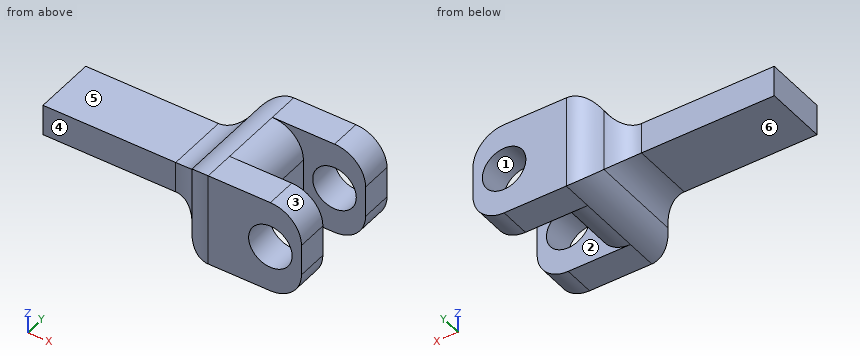
```python
from build123d import *

# Parameters (mm, degrees)
F1_DEPTH = 7.5
F3_D     = 7
F4_R     = 5
F5_R     = 4.99999
F6_W     = 10
F6_H     = 5
F7_DEPTH = 25
F8_R     = 5


# Not quite as in the source:
# - a fillet or chamfer is up to 0.001 mm smaller than in the source, because OpenCascade refuses the exact size


with BuildPart() as f1:
    # F0 (on Top) → F1 (new body, symmetric)
    with BuildSketch(Plane.XY):
        Polygon((10, 10), (-10, 10), (-10, -10), (10, -10), (10, -5), (0, -5), (0, 5), (10, 5), align=None)
    extrude(amount=F1_DEPTH, both=True)

    # F3 (through all)
    with Locations(Plane(origin=(0, 10, 0), x_dir=(-1, 0, 0), z_dir=(0, 1, 0))):
        with Locations((-5, 0)):
            Hole(F3_D / 2)

    # F4
    f4_edges = [f1.edges().sort_by_distance(p)[0] for p in [
        (10, 7.5, 7.5),
        (10, 7.5, -7.5),
        (10, -7.5, 7.5),
        (10, -7.5, -7.5),
        (-10, 10, 0),
        (-10, 0, -7.5),
        (-10, -10, 0),
        (-10, 0, 7.5),
    ]]
    fillet(f4_edges, radius=F4_R)

    # F5 (radius 5 in the source; OpenCascade refuses exactly that, so slightly less here)
    f5_edges = [f1.edges().sort_by_distance(p)[0] for p in [
        (0, 0, 7.5),
        (0, 0, -7.5),
    ]]
    fillet(f5_edges, radius=F5_R)

    # F6 (on face) → F7 (join)
    with BuildSketch(Plane(origin=(-10, 0, 0), x_dir=(0, -1, 0), z_dir=(-1, 0, 0))):
        Rectangle(F6_W, F6_H)
    extrude(amount=F7_DEPTH)

    # F8
    f8_edges = [f1.edges().sort_by_distance(p)[0] for p in [
        (-10, 0, 2.5),
        (-10, -5, 0),
        (-10, 0, -2.5),
        (-10, 5, 0),
    ]]
    fillet(f8_edges, radius=F8_R)


solid = f1.part
```
Here's how the part is built. I have some questions about the finished solid (model axes, mm). Face numbers are marked on the shaded views. A direction names the side the tool comes from. Give positions to 0.01 mm unless a question says otherwise; leave off trailing zeros. Loops run counter-clockwise (first coordinate to the right, second up) from the corner with the lowest first, then second, coordinate; pieces in that order, holes last. Notation, with made-up numbers: M 55,66 L 103,66 A36 ccw 103,103 Z; hole C 25,-18.5 d10. An arc over 180 degrees is marked long. Put each result on its own line as item: value. Start each with the question number.
(1) If we mould it in two halves opening along Z, with no side actions, what happens to the marked faces 1, 2 and 3? For each: +Z half, -Z half, draft (parallel to the pull), parting line (faces both ways), or undercut.
(2) I want a section at A-A on z = 0. Please give me the cut outline in (x, y).
(3) I need wall thicknesses on line 1 along Y through (x, z) = (2, 4.25); line 2 along X through (y, z) = (-4.5, 1); line 3 along Z through (x, y) = (-27, -2). Which ranges of each line are inside material? Lowest first, please. Write a range as [from, to].
(4) For the marked faces 4, 5 and 6, which set-ups out of +Z, -Z, +X, -X, +Y, -Y let a thin tool reach every point of the face, with its end or its side?
(5) I want a section at B-B on x = 2. Please give me the cut outline in (y, z), then the cut area to 3 significant figures.
(6) Will these pins go through, and if not, where does the flat tip stop? pin 1 Ø3 at (x, y) = (-28, 2) entering from +Z; pin 2 Ø6 at (x, y) = (-9, 4.5) entering from +Z; pin 3 Ø8 at (x, z) = (-24.5, 2.5) entering from -Y; pin 4 Ø5.5 at (x, z) = (5, 0) entering from +Y.
(7) I want a section at C-C on y = -7. Please give me the cut outline in (x, z), then the cut area to 3 significant figures.
Answer block:
1. face 1: undercut
1. face 2: draft
1. face 3: +Z half
2. outline: M -35,-5 L -13.66,-5 A5 cw -9.33,-7.5 A5 ccw -5,-10 L 1.5,-10 L 1.5,-5 L 0,-5 L 0,5 L 1.5,5 L 1.5,10 L -5,10 A5 ccw -9.33,7.5 A5 cw -13.66,5 L -35,5 Z; M 8.5,-10 L 10,-10 L 10,-5 L 8.5,-5 Z; M 8.5,5 L 10,5 L 10,10 L 8.5,10 Z
3. line 1: [-10, -5], [5, 10]
3. line 2: [-35, 0]
3. line 3: [-2.5, 2.5]
4. face 4: +Z, -Z, -X, -Y
4. face 5: +Z, -X, +Y, -Y
4. face 6: -Z, -X, +Y, -Y
5. outline: M -10,-7.5 L -5,-7.5 L -5,-1.8 L -10,-1.8 Z; M -10,1.8 L -5,1.8 L -5,7.5 L -10,7.5 Z; M 5,-7.5 L 10,-7.5 L 10,-1.8 L 5,-1.8 Z; M 5,1.8 L 10,1.8 L 10,7.5 L 5,7.5 Z
5. area: 114 mm^2
6. pin 1: z = 2.5
6. pin 2: z = 7.4
6. pin 3: y = -5
6. pin 4: through
7. outline: M -9.66,-4.5 A5 cw -9.33,-5 A5 ccw -5,-7.5 L 5,-7.5 A5 ccw 10,-2.5 L 10,2.5 A5 ccw 5,7.5 L -5,7.5 A5 ccw -9.33,5 A5 cw -9.66,4.5 Z; hole C 5,0 d7
7. area: 238 mm^2
